Geometry check sheet. Reference: the model listing, model coordinates, mm. Face numbers are marked on the shaded views. A direction names the side the tool comes from. Round coordinates to 2 decimals unless told otherwise and drop trailing zeros. Loops run counter-clockwise (first coordinate to the right, second up) from the corner with the lowest first, then second, coordinate; pieces in that order, holes last.
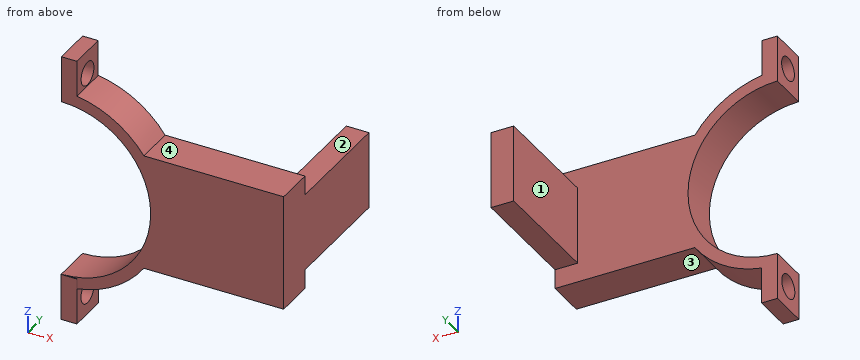
```python
from build123d import *

# Parameters (mm, degrees)
F1_DEPTH      = 5
F2_R          = 11.5
F3_DEPTH      = 25
F4_W          = 19.7234917432
F4_H          = 22.7468013763
F5_DEPTH      = 20.501
F5_DEPTH_BACK = 50
F7_START      = 4
F6_W          = 2.0386253018
F6_H          = 5.0671915524
F7_DEPTH      = 6
F8_R          = 1.5364131309
F9_DEPTH      = 25
F10_W         = 2.9216879989
F10_H         = 10
F11_DEPTH     = 15
F13_START     = 4
F12_W         = 2
F12_H         = 5
F13_DEPTH     = 6
F14_R         = 1.5
F15_DEPTH     = 25


with BuildPart() as f1:
    # F0 (on Front) → F1 (new body)
    with BuildSketch(Plane.XZ):
        with BuildLine():
            Line((10.6183802908, -7.5), (28.6183802908, -7.5))
            Line((28.6183802908, -7.5), (28.6183802908, 7.5))
            Line((28.6183802908, 7.5), (10.6183802908, 7.5))
            ThreePointArc((10.6183802908, 7.5), (-13, 0), (10.6183802908, -7.5))
        make_face()
    extrude(amount=F1_DEPTH)

    # F2 (on face) → F3 (cut)
    with BuildSketch(Plane.XZ.offset(5)):
        Circle(F2_R)
    extrude(amount=-F3_DEPTH, mode=Mode.SUBTRACT)

    # F4 (on face) → F5 (cut, two sides)
    with BuildSketch(Plane(origin=(0, 0, -7.5), x_dir=(1, 0, 0), z_dir=(0, 0, -1))) as f5_sk:
        with Locations((-9.8617458716, 1.8715718761)):
            Rectangle(F4_W, F4_H)
    extrude(amount=-F5_DEPTH, mode=Mode.SUBTRACT)
    extrude(f5_sk.sketch, amount=F5_DEPTH_BACK, mode=Mode.SUBTRACT)

    # F6 (on face) → F7 (join)
    with BuildSketch(Plane(origin=(0, 0, -7.5), x_dir=(1, 0, 0), z_dir=(0, 0, -1)).offset(F7_START)):
        with Locations((1.0193126509, 2.5335957762)):
            Rectangle(F6_W, F6_H)
    extrude(amount=F7_DEPTH)

    # F8 (on face) → F9 (cut)
    with BuildSketch(Plane(origin=(0, 0, 0), x_dir=(0, -1, 0), z_dir=(-1, 0, 0))):
        with Locations((2.5671915524, -14.5)):
            Circle(F8_R)
    extrude(amount=-F9_DEPTH, mode=Mode.SUBTRACT)

    # F10 (on face) → F11 (join)
    with BuildSketch(Plane(origin=(0, 0, 0), x_dir=(-1, 0, 0), z_dir=(0, 1, 0))):
        with Locations((-27.1575362913, 0)):
            Rectangle(F10_W, F10_H)
    extrude(amount=F11_DEPTH)

    # F12 (on face) → F13 (join)
    with BuildSketch(Plane.XY.offset(7.5).offset(F13_START)):
        with Locations((1, -2.5)):
            Rectangle(F12_W, F12_H)
    extrude(amount=F13_DEPTH)

    # F14 (on face) → F15 (cut)
    with BuildSketch(Plane(origin=(0, 0, 0), x_dir=(0, -1, 0), z_dir=(-1, 0, 0))):
        with Locations((2.5, 14.5)):
            Circle(F14_R)
    extrude(amount=-F15_DEPTH, mode=Mode.SUBTRACT)


solid = f1.part
```
1) Gauge pin test, flat ends, axial feed: pin 1 (5 mm diameter, centred on y = -2, z = 15.5, fed in from +X); pin 2 (1.5 mm diameter, centred on x = 27, y = 5.5, fed in from -Z); pin 3 (5.5 mm diameter, centred on x = 18, y = -3.5, fed in from -Z); pin 4 (3 mm diameter, centred on y = -0.5, z = -13.5, fed in from -X). Record the tip position at first contact, or that the pin passes through.
Report:
pin 1: stops at x = 2
pin 2: stops at z = -5
pin 3: stops at z = -7.5
pin 4: stops at x = 0
2) Sectioned sample at D-D, the plane z = 0. Record the cut outline in (x, y).
Report:
outline: (11.5, -5) - (28.62, -5) - (28.62, 15) - (25.7, 15) - (25.7, 0) - (11.5, 0) - close
3) Sectioned sample at C-C, the plane x = 7.75. Record the cut outline in (y, z), then the cut area to 3 significant figures.
Report:
outline: (-5, -10.44) - (0, -10.44) - (0, -8.5) - (-5, -8.5) - close; (-5, 8.5) - (0, 8.5) - (0, 10.44) - (-5, 10.44) - close
area: 19.4 mm2
4) Access from +Z, -Z, +X, -X, +Y, -Y to the whole of each face (thin tool, end or side, straight path). Record for the marked faces 1, 2, 3 and 4.
Report:
face 1: +Z, -Z, -X, +Y
face 2: +Z, +X, -X, +Y
face 3: -Z, +X, +Y, -Y
face 4: +Z, +X, +Y, -Y
5) Sectioned sample at B-B, the plane y = -2.5. Record the cut outline in (x, z), then the cut area to 3 significant figures.
Report:
outline: (0, -17.5) - (2.04, -17.5) - (2.04, -16.03) - (0, -16.03) - close; (0, -12.97) - (2.04, -12.97) - (2.04, -12.84) arc R13 ccw to (10.62, -7.5) - (28.62, -7.5) - (28.62, 7.5) - (10.62, 7.5) arc R13 ccw to (2, 12.85) - (2, 13) - (0, 13) - (0, 11.5) arc R11.5 cw to (0, -11.5) - close; (0, 16) - (2, 16) - (2, 17.5) - (0, 17.5) - close
area: 310 mm2
6) Scan lines: line 1 along Z through (x, y) = (1.15, -2.5); line 2 along Z through (x, y) = (0.95, -2.5); line 3 along X through (y, z) = (3.5, 1.5). Record each from-to range of solid material in increasing order.
Report:
line 1: z = -17.5 to -16.03, -12.97 to -11.44, 11.44 to 13, 16 to 17.5
line 2: z = -17.5 to -16.03, -12.97 to -11.46, 11.46 to 13, 16 to 17.5
line 3: x = 25.7 to 28.62
7) Sectioned sample at A-A, the plane z = 14.5. Record the cut outline in (x, y), then the cut area to 3 significant figures.
Report:
outline: (0, -5) - (2, -5) - (2, -4) - (0, -4) - close; (0, -1) - (2, -1) - (2, 0) - (0, 0) - close
area: 4.00 mm2
